Part model, mm, in its own coordinate system. A direction names the side the tool comes from. Give positions to 0.01 mm unless a question says otherwise; leave off trailing zeros. Order: outer loops, then holes, each group sorted by start corner. A loop starts at its lowest first (then second) coordinate and runs counter-clockwise, first axis right, second up. Notation, with made-up numbers: (69, -19) -> (119, -19) arc R11 ccw to (119, 2) -> close; hole circle Ø11 at (48, 7). An arc over 180 degrees is marked (long way). Write item = value, one per line. Start each with the question number.
Item 1: Band-saw the part on A-A on z = -115. Write the cut outline in (x, y) (3 decimals).
Item 2: Band-saw the part on B-B on y = 0. Write the cut outline in (x, z) (3 decimals).
Item 3: Flat gauge pins, fed straight in: P1, Ø1, axis at x = 6, y = 23.5, coming from the +Z side; P2, Ø2.5, axis at x = -6, y = 24.5, coming from the +Z side; P3, Ø18, axis at y = 0, z = 0, coming from the -X side; P4, Ø2.5, axis at x = -8.5, y = -24, coming from the +Z side. Where does each tip first touch, or does it go through?
Item 4: Drill centre lines: line 1 along X through (y, z) = (6, -26) (3 decimals); line 2 along X through (y, z) = (20.5, -49.5) (3 decimals). Where is each one in solid material? Low to high.
Item 5: Tool access for faces 1 (the face through (-22.225, -10, 4)), 2 (the face through (0, -25.4, 4)): list every direction of +Z, -Z, +X, -X, +Y, -Y with a clear straight run to the whole face (end or side of a thin tool).
Item 6: Pull direction Z, two halves, no side cores. Call faces 3 (the face through (0, -22.225, 4)), 4 (the face through (-23.835, -9.685, -2.151)), 5 (the face through (22.5, -0.1, 228.7)): +Z half, -Z half, draft (parallel to the pull), parting line (faces both ways), or undercut.
Item 7: Band-saw the part on C-C on z = 0. Write the cut outline in (x, y) (3 decimals).
```python
from build123d import *

# Parameters (mm, degrees)
SKETCH1_W                   = 50.8
SKETCH1_H                   = 50.8
SKETCH1_W_2                 = 44.45
SKETCH1_H_2                 = 44.45
BOSS_EXTRUDE1_DEPTH         = 254
FILLET1_R                   = 6.35
CUT_EXTRUDE1_DEPTH          = 914.4
F_1_4_START                 = -25.4
F_1_4_CLEARANCE_SLOT1_DEPTH = 50.8
F_3_4_CLEARANCE_HOLE1_D     = 19.84248


# Read off the part's stored shape, not the designer's step: 1/4 Clearance Slot1
with BuildPart() as part:
    # Sketch1 → Boss-Extrude1 (new, symmetric)
    with BuildSketch(Plane.XY):
        Rectangle(SKETCH1_W, SKETCH1_H)
        Rectangle(SKETCH1_W_2, SKETCH1_H_2, mode=Mode.SUBTRACT)
    extrude(amount=BOSS_EXTRUDE1_DEPTH, both=True)

    # Fillet1
    fillet1_edges = [part.edges().sort_by_distance(p)[0] for p in [
        (-25.4, 25.4, 0),
        (25.4, 25.4, 0),
        (25.4, -25.4, 0),
        (-25.4, -25.4, 0),
    ]]
    fillet(fillet1_edges, radius=FILLET1_R)

    # Sketch2 → Cut-Extrude1 (cut)
    with BuildSketch(Plane.ZY.offset(25.4)):
        Polygon((254, -25.4), (203.2, 25.4), (254, 25.4), align=None)
        Polygon((-254, 25.4), (-254, -25.4), (-203.2, 25.4), align=None)
    extrude(amount=-CUT_EXTRUDE1_DEPTH, mode=Mode.SUBTRACT)

    # 1/4 Clearance Slot1 outline → 1/4 Clearance Slot1 (cut)
    with BuildSketch(Plane(origin=(0, 0, 0), x_dir=(1, 0, 0), z_dir=(0, 1, 0)).offset(F_1_4_START)):
        with BuildLine():
            ThreePointArc((-0.88265, -47.7139), (2.38125, -44.45), (-0.88265, -41.1861))
            Line((-0.88265, -41.1861), (-11.81735, -41.1861))
            ThreePointArc((-11.81735, -41.1861), (-15.08125, -44.45), (-11.81735, -47.7139))
            Line((-11.81735, -47.7139), (-0.88265, -47.7139))
        make_face()
        with BuildLine():
            ThreePointArc((11.81735, -31.8389), (15.08125, -28.575), (11.81735, -25.3111))
            Line((11.81735, -25.3111), (0.88265, -25.3111))
            ThreePointArc((0.88265, -25.3111), (-2.38125, -28.575), (0.88265, -31.8389))
            Line((0.88265, -31.8389), (11.81735, -31.8389))
        make_face()
        with BuildLine():
            ThreePointArc((-0.88265, 25.3111), (2.38125, 28.575), (-0.88265, 31.8389))
            Line((-0.88265, 31.8389), (-11.81735, 31.8389))
            ThreePointArc((-11.81735, 31.8389), (-15.08125, 28.575), (-11.81735, 25.3111))
            Line((-11.81735, 25.3111), (-0.88265, 25.3111))
        make_face()
        with BuildLine():
            Line((0.88265, 41.1861), (11.81735, 41.1861))
            ThreePointArc((11.81735, 41.1861), (15.08125, 44.45), (11.81735, 47.7139))
            Line((11.81735, 47.7139), (0.88265, 47.7139))
            ThreePointArc((0.88265, 47.7139), (-2.38125, 44.45), (0.88265, 41.1861))
        make_face()
    extrude(amount=F_1_4_CLEARANCE_SLOT1_DEPTH, mode=Mode.SUBTRACT)

    # 3/4 Clearance Hole1 (through all)
    with Locations(Plane(origin=(25.4, 0, 0), x_dir=(0, 0, -1), z_dir=(1, 0, 0))):
        with Locations((0, 0)):
            Hole(F_3_4_CLEARANCE_HOLE1_D / 2)


solid = part.part
```
Values found:
q1.outline = (-25.4, -19.05) arc R6.35 ccw to (-19.05, -25.4) -> (19.05, -25.4) arc R6.35 ccw to (25.4, -19.05) -> (25.4, 19.05) arc R6.35 ccw to (19.05, 25.4) -> (-19.05, 25.4) arc R6.35 ccw to (-25.4, 19.05) -> close; hole (-22.225, -22.225) -> (22.225, -22.225) -> (22.225, 22.225) -> (-22.225, 22.225) -> close
q2.outline = (-25.4, -228.6) -> (-22.225, -228.6) -> (-22.225, -9.921) -> (-25.4, -9.921) -> close; (-25.4, 9.921) -> (-22.225, 9.921) -> (-22.225, 228.6) -> (-25.4, 228.6) -> close; (22.225, -228.6) -> (25.4, -228.6) -> (25.4, -9.921) -> (22.225, -9.921) -> close; (22.225, 9.921) -> (25.4, 9.921) -> (25.4, 228.6) -> (22.225, 228.6) -> close
q3.P1 = 205.6
q3.P2 = 205.35
q3.P3 = through
q3.P4 = 253.85
q4.line_1 = -25.4 to -22.225, 22.225 to 25.4
q4.line_2 = -25.232 to -22.225, 22.225 to 25.232
q5.face_1 = +Z, -Z
q5.face_2 = +Z, -Z, +X, -X, -Y
q6.face_3 = draft
q6.face_4 = undercut
q6.face_5 = +Z half
q7.outline = (-25.4, -19.05) arc R6.35 ccw to (-19.05, -25.4) -> (19.05, -25.4) arc R6.35 ccw to (25.4, -19.05) -> (25.4, -9.921) -> (22.225, -9.921) -> (22.225, -22.225) -> (-22.225, -22.225) -> (-22.225, -9.921) -> (-25.4, -9.921) -> close; (-25.4, 9.921) -> (-22.225, 9.921) -> (-22.225, 22.225) -> (22.225, 22.225) -> (22.225, 9.921) -> (25.4, 9.921) -> (25.4, 19.05) arc R6.35 ccw to (19.05, 25.4) -> (-19.05, 25.4) arc R6.35 ccw to (-25.4, 19.05) -> close
